Design review of the part built by this model. Coordinates are the model's own, in mm. Face numbers are marked on the shaded views. A direction names the side the tool comes from. Give positions to 0.01 mm unless a question says otherwise; leave off trailing zeros. Write each loop counter-clockwise with the first axis right and the second up, starting at its lowest first coordinate (ties: lowest second). Pieces come first, ordered by that corner, then holes.
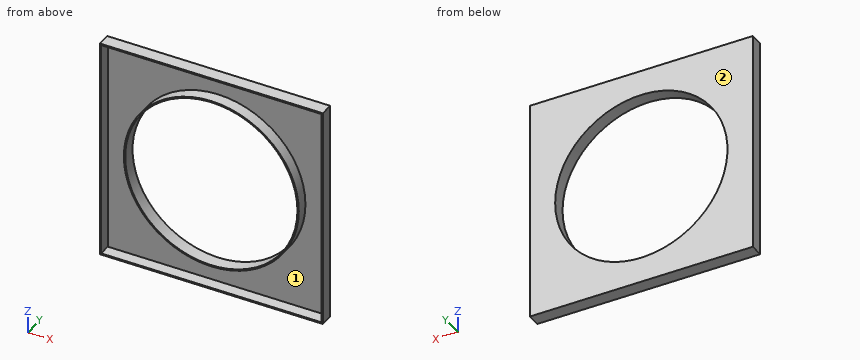
```python
from build123d import *

# Parameters (mm, degrees)
F0_W     = 420
F0_H     = 420
F0_R     = 162.300497
F1_DEPTH = 25
F2_DEPTH = 25
F3_T     = -2.5


with BuildPart() as f1:
    # F0 (on Front) → F1 (new body)
    with BuildSketch(Plane.XZ):
        Rectangle(F0_W, F0_H)
        Circle(F0_R, mode=Mode.SUBTRACT)
    extrude(amount=F1_DEPTH)

    # F0 (on Front) → F2 (join)
    with BuildSketch(Plane.XZ):
        Rectangle(F0_W, F0_H)
        Circle(F0_R, mode=Mode.SUBTRACT)
    extrude(amount=F2_DEPTH)

    # F3
    f3_openings = [f1.faces().sort_by_distance(p)[0] for p in [
        (-204.060303, -25, 0),
    ]]
    offset(amount=F3_T, openings=f3_openings)


solid = f1.part
```
(1) Consider section B-B, the plane x = 0. Give the boundary of the cut face in (y, z).
Resolved:
outline: (-25, -210) - (0, -210) - (0, -162.3) - (-25, -162.3) - (-25, -164.8) - (-2.5, -164.8) - (-2.5, -207.5) - (-25, -207.5) - close; (-25, 162.3) - (0, 162.3) - (0, 210) - (-25, 210) - (-25, 207.5) - (-2.5, 207.5) - (-2.5, 164.8) - (-25, 164.8) - close
(2) Consider section C-C, the plane z = 0. Give the boundary of the cut face in (x, y), then the cut area to 3 significant figures.
Resolved:
outline: (-210, -25) - (-207.5, -25) - (-207.5, -2.5) - (-164.8, -2.5) - (-164.8, -25) - (-162.3, -25) - (-162.3, 0) - (-210, 0) - close; (162.3, -25) - (164.8, -25) - (164.8, -2.5) - (207.5, -2.5) - (207.5, -25) - (210, -25) - (210, 0) - (162.3, 0) - close
area: 463 mm2
(3) To check wall thickness, follow L1, parallel to X at y = -5, z = 3; L2, parallel to Z at x = 0, y = -12.5; L3, parallel to X at y = -10.5, z = -121.5. State the ranges of each line that lie inside material, in increasing order.
Resolved:
L1: x = -210 to -207.5, -164.77 to -162.27, 162.27 to 164.77, 207.5 to 210
L2: z = -210 to -207.5, -164.8 to -162.3, 162.3 to 164.8, 207.5 to 210
L3: x = -210 to -207.5, -111.34 to -107.61, 107.61 to 111.34, 207.5 to 210
(4) Tool access review of the marked faces 1 and 2: name each direction out of +Z, -Z, +X, -X, +Y, -Y from which nothing blocks a thin tool from reaching the whole face with its end or side.
Resolved:
face 1: -Y
face 2: +Z, -Z, +X, -X, +Y
(5) Consider section D-D, the plane z = -183. Give the boundary of the cut face in (x, y), then the cut area to 3 significant figures.
Resolved:
outline: (-210, -25) - (-207.5, -25) - (-207.5, -2.5) - (207.5, -2.5) - (207.5, -25) - (210, -25) - (210, 0) - (-210, 0) - close
area: 1,160 mm2
(6) Consider section A-A, the plane y = -20. Give the boundary of the cut face in (x, z).
Resolved:
outline: (-210, -210) - (210, -210) - (210, 210) - (-210, 210) - close; circle Ø329.6 at (0, 0); hole (-207.5, -207.5) - (207.5, -207.5) - (207.5, 207.5) - (-207.5, 207.5) - close; hole circle Ø324.6 at (0, 0)
